from build123d import *

# Parameters (mm, degrees)
SKETCH1_W           = 36.957
SKETCH1_H           = 21.3995
SKETCH1_R           = 0.9525
BOSS_EXTRUDE1_DEPTH = 2.38125
CUT_EXTRUDE1_REACH  = 4.381
SKETCH2_W           = 19.05
SKETCH2_H           = 15.8115


with BuildPart() as part:
    # Sketch1 → Boss-Extrude1 (new body)
    with BuildSketch(Plane.XY):
        with Locations((16.891, 9.11225)):
            Rectangle(SKETCH1_W, SKETCH1_H)
        with Locations((1.5875, 14.25575)):
            Circle(SKETCH1_R, mode=Mode.SUBTRACT)
        with Locations((32.1945, 1.5875)):
            Circle(SKETCH1_R, mode=Mode.SUBTRACT)
    extrude(amount=BOSS_EXTRUDE1_DEPTH)

    # Sketch2 → Cut-Extrude1 (cut, up to next)
    with BuildSketch(Plane.XY.offset(2.38125), mode=Mode.PRIVATE) as cut_extrude1_sk1:
        with Locations((16.891, 6.31825)):
            Rectangle(SKETCH2_W, SKETCH2_H)
    cut_extrude1_tool1 = extrude(cut_extrude1_sk1.sketch, amount=-CUT_EXTRUDE1_REACH, mode=Mode.PRIVATE) & part.part
    add(cut_extrude1_tool1.solids().sort_by_distance((16.891, 6.31825, 2.38125))[0], mode=Mode.SUBTRACT)


solid = part.part
The model under review builds one solid part; all positions refer to its coordinate system, in mm. A direction names the side the tool comes from. Coordinates: 2 decimals unless noted, no trailing zeros. Order: outer loops, then holes, each group sorted by start corner. A loop starts at its lowest first (then second) coordinate and runs counter-clockwise, first axis right, second up. Notation, with made-up numbers: (-24, 74) -> (33, 74) arc R16 ccw to (33, 96) -> close; hole circle Ø10 at (79.5, -23.75). An arc over 180 degrees is marked (long way). Answer in a Markdown table with one row per item.
(1) The part is to be moulded in two halves that separate along Y. For faces 1 (the cylindrical face through (0.636, 14.298, 1.174)), 2 (the flat face through (35.37, 9, 1)), 3 (the cylindrical face through (33.074, 1.223, 1.174)), 4 (the flat face through (31, -1.588, 1)), say which applies: +Y half, -Y half, draft (parallel to the pull), parting line (faces both ways), or undercut.
Answers:
| item | result |
|---|---|
| face 1 | undercut |
| face 2 | draft |
| face 3 | undercut |
| face 4 | -Y half |
(2) Consider section B-B (x = 25). Write out the cut boundary in (y, z).
Answers:
| item | result |
|---|---|
| outline | (14.22, 0) -> (19.81, 0) -> (19.81, 2.38) -> (14.22, 2.38) -> close |
(3) Consider section C-C (z = 1.2). Write out the cut boundary in (x, y) (1 decimal).
Answers:
| item | result |
|---|---|
| outline | (-1.6, -1.6) -> (7.4, -1.6) -> (7.4, 14.2) -> (26.4, 14.2) -> (26.4, -1.6) -> (35.4, -1.6) -> (35.4, 19.8) -> (-1.6, 19.8) -> close; hole circle Ø1.9 at (1.6, 14.3); hole circle Ø1.9 at (32.2, 1.6) |
(4) Machinability: for faces 5 (the flat face through (17, 16, 0)), 6 (the flat face through (7.366, 6, 1)), which of the approach directions +Z, -Z, +X, -X, +Y, -Y give a long, thin tool a straight path to every point of the face, cutting with its end or side? Answer none if there is none.
Answers:
| item | result |
|---|---|
| face 5 | -Z, +X, -X, +Y, -Y |
| face 6 | +Z, -Z, -Y |
(5) Wall thickness on line 1 along X through (y, z) = (10.75, 0.9); line 2 along X through (y, z) = (1.75, 1); line 3 along Y through (x, z) = (21.5, 1.9): over which ranges is each line inside the solid? List them lowest first.
Answers:
| item | result |
|---|---|
| line 1 | -1.59 to 7.37, 26.42 to 35.37 |
| line 2 | -1.59 to 7.37, 26.42 to 31.26, 33.13 to 35.37 |
| line 3 | 14.22 to 19.81 |
(6) Insertion check: pin 1 (6 mm diameter, centred on x = 15, y = 17, fed in from -Z); pin 2 (0.7 mm diameter, centred on x = 20.5, z = 1.5, fed in from -Y). Each pin has a flat end and moves straight along its axis. Give the tip position at first contact, or say it passes through.
Answers:
| item | result |
|---|---|
| pin 1 | z = 0 |
| pin 2 | y = 14.22 |
(7) Consider section A-A (y = 0). Write out the cut boundary in (x, z), plus the area to 3 significant figures.
Answers:
| item | result |
|---|---|
| outline | (-1.59, 0) -> (7.37, 0) -> (7.37, 2.38) -> (-1.59, 2.38) -> close; (26.42, 0) -> (35.37, 0) -> (35.37, 2.38) -> (26.42, 2.38) -> close |
| area | 42.6 mm² |
